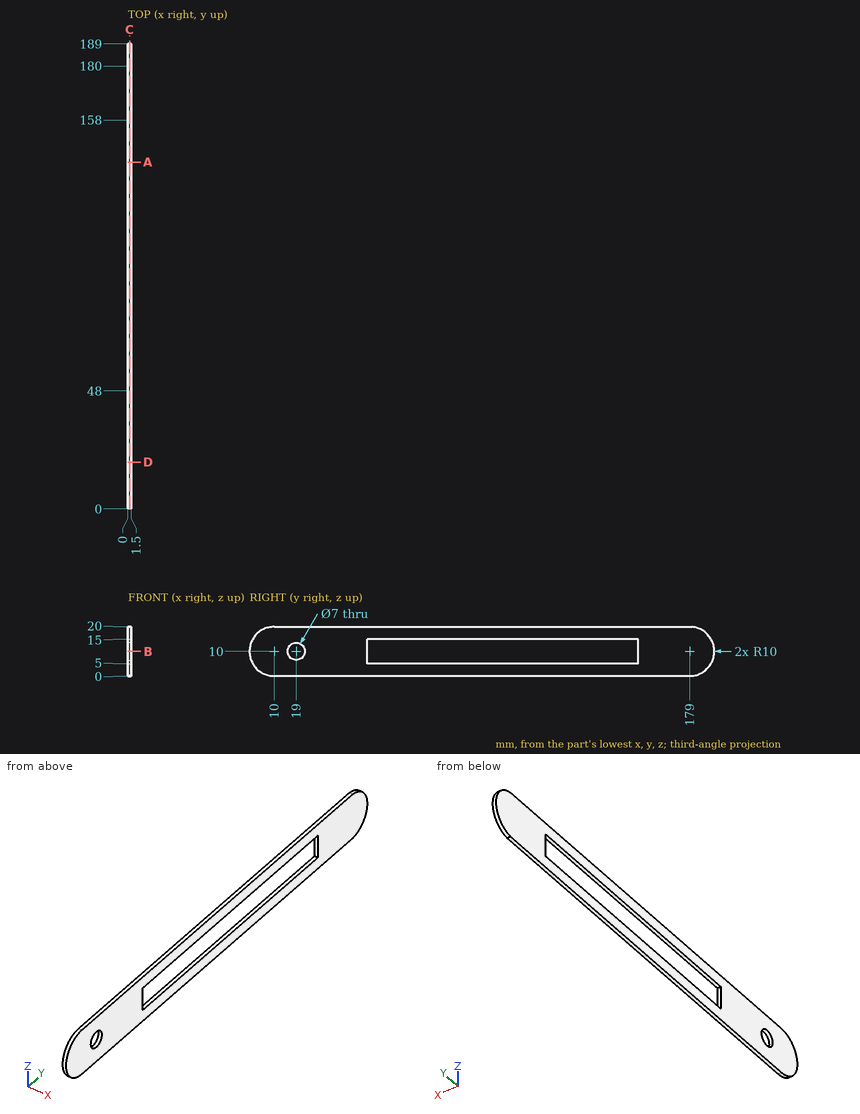
Print and shaded views of the part. All mm, measured from the part's lowest x, y and z. Round coordinates to 2 decimals unless told otherwise and drop trailing zeros. Write each loop counter-clockwise with the first axis right and the second up, starting at its lowest first coordinate (ties: lowest second). Pieces come first, ordered by that corner, then holes. Notation, with made-up numbers: (12.25, 79) - (44.25, 79) arc R13 ccw to (44.25, 91) - close; hole circle Ø6 at (75, 87.25). An arc over 180 degrees is marked (long way). Write each question's results on one line, items separated by ' | '. Start each with the question number.
Item 1: Saw through at D-D (y = 19). Write the cut outline in (x, z).
Item 2: Saw through at A-A (y = 141). Write the cut outline in (x, z), and give its area (3 significant figures).
Item 3: Wall check: L1, parallel to Y at x = 1, z = 10; L2, parallel to Z at x = 0.7, y = 139; L3, parallel to Z at x = 0.85, y = 19. Give the ranges that are in metal, low to high. Write a range as [from, to].
Item 4: Saw through at B-B (z = 10). Write the cut outline in (x, y).
Item 5: Saw through at C-C (x = 0.8). Write the cut outline in (y, z).
Item 6: Drop a flat-ended pin along its axis: P1, Ø4, axis at y = 19, z = 10, coming from the +X side. Give the stop position or say it passes through.
Results are:
1) outline: (0, 0) - (1.5, 0) - (1.5, 6.5) - (0, 6.5) - close; (0, 13.5) - (1.5, 13.5) - (1.5, 20) - (0, 20) - close
2) outline: (0, 0) - (1.5, 0) - (1.5, 5) - (0, 5) - close; (0, 15) - (1.5, 15) - (1.5, 20) - (0, 20) - close | area: 15.0 mm²
3) L1: y = [0, 15.5], [22.5, 48], [158, 189] | L2: z = [0, 5], [15, 20] | L3: z = [0, 6.5], [13.5, 20]
4) outline: (0, 0) - (1.5, 0) - (1.5, 15.5) - (0, 15.5) - close; (0, 22.5) - (1.5, 22.5) - (1.5, 48) - (0, 48) - close; (0, 158) - (1.5, 158) - (1.5, 189) - (0, 189) - close
5) outline: (10, 0) - (180, 0) - (180, 0.05) arc R10 ccw to (180, 19.95) - (180, 20) - (10, 20) arc R10 ccw to start; hole circle Ø7 at (19, 10); hole (48, 5) - (158, 5) - (158, 15) - (48, 15) - close
6) P1: passes through
